Check sheet for the modelled part. Datum: model origin and axes. Units: mm. A direction names the side the tool comes from. Round coordinates to 2 decimals unless told otherwise and drop trailing zeros. Write each loop counter-clockwise with the first axis right and the second up, starting at its lowest first coordinate (ties: lowest second). Pieces come first, ordered by that corner, then holes. Notation, with made-up numbers: (25.5, 5.25) -> (55.5, 5.25) arc R14 ccw to (55.5, 23.25) -> close; hole circle Ø11 at (80, -13.75). An arc over 180 degrees is marked (long way). One line per item, written item: value.
from build123d import *

# Parameters (mm, degrees)
F0_R     = 8
F1_DEPTH = 3.5
F2_R     = 12.5
F3_DEPTH = 1
F4_W     = 20
F4_H     = 2
F5_DEPTH = 2


with BuildPart() as f1:
    # F0 (on Top) → F1 (new body)
    with BuildSketch(Plane.XY):
        with BuildLine():
            ThreePointArc((0, -12.5), (-12.5, 0), (0, 12.5))
            Line((0, 12.5), (-35, 12.5))
            Line((-35, 12.5), (-116.388784, 2.506714))
            Line((-116.388784, 2.506714), (-116.388784, -2.506714))
            Line((-116.388784, -2.506714), (-35, -12.5))
            Line((-35, -12.5), (0, -12.5))
        make_face()
        with BuildLine():
            ThreePointArc((0, -12.5), (8.838835, -8.838835), (12.5, 0))
            ThreePointArc((12.5, 0), (8.838835, 8.838835), (0, 12.5))
            ThreePointArc((0, 12.5), (-12.5, 0), (0, -12.5))
        make_face()
        Circle(F0_R, mode=Mode.SUBTRACT)
    extrude(amount=F1_DEPTH)

    # F2 (on face) → F3 (join)
    with BuildSketch(Plane.XY.offset(3.5)):
        Circle(F2_R)
    extrude(amount=F3_DEPTH)

    # F4 (on face) → F5 (cut)
    with BuildSketch(Plane.XY.offset(3.5)):
        with Locations((-106.388784, 0.006714)):
            Rectangle(F4_W, F4_H)
    extrude(amount=-F5_DEPTH, mode=Mode.SUBTRACT)


solid = f1.part
Item 1: Sectioned sample at C-C on x = -31. Enter the section's corners in (y, z).
Answer:
outline: (-12.5, 0) -> (12.5, 0) -> (12.5, 3.5) -> (-12.5, 3.5) -> close
Item 2: Sectioned sample at A-A on y = 6.75. Enter the section's corners in (x, z), and give its area (3 significant figures).
Answer:
outline: (-81.83, 0) -> (-4.29, 0) -> (-4.29, 3.5) -> (4.29, 3.5) -> (4.29, 0) -> (10.52, 0) -> (10.52, 4.5) -> (-10.52, 4.5) -> (-10.52, 3.5) -> (-81.83, 3.5) -> close
area: 314 mm^2
Item 3: Sectioned sample at D-D on x = -55. Enter the section's corners in (y, z).
Answer:
outline: (-10.04, 0) -> (10.04, 0) -> (10.04, 3.5) -> (-10.04, 3.5) -> close
Item 4: Tool access check on faces 4 (the flat face through (-107, 0, 1.5)), 5 (the cylindrical face through (-1.73, -7.81, 1.73)), 6 (the flat face through (-75.125, 7.573, 1.726)). Record the directions out of +Z, -Z, +X, -X, +Y, -Y that give a thin tool (end or side, any length) a straight path to the whole face; none if there is none.
Answer:
face 4: +Z, -X
face 5: -Z
face 6: +Z, -Z, -X, +Y
Item 5: Mould release check, pull along X, two halves, no side actions. Record for faces 1 (the flat face through (0, 0, 3.5)), 2 (the flat face through (-96.389, 0, 3)), 3 (the flat face through (0, 0, 4.5)): pulls with the +X half, pulls with the -X half, needs draft (parallel to the pull), parting line crosses it, or undercut.
Answer:
face 1: undercut
face 2: pulls with the -X half
face 3: needs draft
Item 6: Sectioned sample at B-B on x = -102.5. Enter the section's corners in (y, z).
Answer:
outline: (-4.21, 0) -> (4.21, 0) -> (4.21, 3.5) -> (1.01, 3.5) -> (1.01, 1.5) -> (-0.99, 1.5) -> (-0.99, 3.5) -> (-4.21, 3.5) -> close
Item 7: Depth check by flat-ended pin: P1, Ø2, axis at x = -103, z = 4, coming from the -Y side; P2, Ø12.5, axis at x = -37, y = -5, coming from the +Z side; P3, Ø0.6, axis at x = -102.5, y = 0, coming from the +Z side. Enter the tip coordinate at first touch or a pass-through.
Answer:
P1: stops at y = -4.26
P2: stops at z = 3.5
P3: stops at z = 1.5
Item 8: Thickness scan on line 1 (Y direction, x = 0, z = 0.85); line 2 (Z direction, x = -71, y = 2.5); line 3 (Y direction, x = -103.5, z = 2.2). Record the ranges inside material, lowest first.
Answer:
line 1: y = -12.5 to -8, 8 to 12.5
line 2: z = 0 to 3.5
line 3: y = -4.09 to -0.99, 1.01 to 4.09
